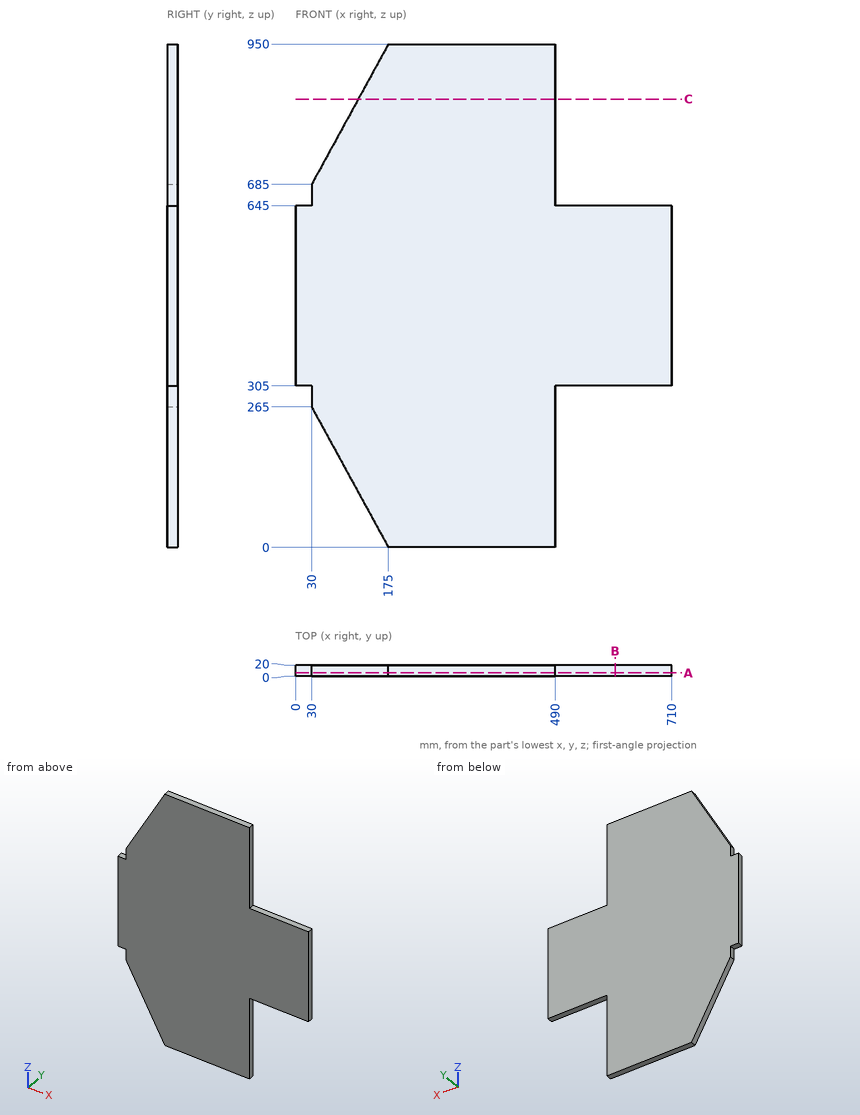
Geometry check sheet. Reference: drawing and pictorial views, mm from the part's lowest x, y, z. Give positions to 0.01 mm unless a question says otherwise; leave off trailing zeros. Write each loop counter-clockwise with the first axis right and the second up, starting at its lowest first coordinate (ties: lowest second). Pieces come first, ordered by that corner, then holes. Notation, with made-up numbers: (58, -35) - (89, -35) arc R16 cw to (89, -9) - close; hole circle Ø4 at (89, -12). An arc over 180 degrees is marked (long way). Use a Markdown table: item, result.
Q1. Section check A-A, the plane y = 6. Enter the section's corners in (x, z), then the cut area to 3 significant figures.
Computed:
| item | result |
|---|---|
| outline | (0, 305) - (30, 305) - (30, 265) - (175, 0) - (490, 0) - (490, 305) - (710, 305) - (710, 645) - (490, 645) - (490, 950) - (175, 950) - (30, 685) - (30, 645) - (0, 645) - close |
| area | 484,000 mm² |
Q2. Section check C-C, the plane z = 846. Enter the section's corners in (x, y), then the cut area to 3 significant figures.
Computed:
| item | result |
|---|---|
| outline | (118.09, 0) - (490, 0) - (490, 20) - (118.09, 20) - close |
| area | 7,440 mm² |
Q3. Thickness scan on L1, parallel to X at y = 5.75, z = 301; L2, parallel to Z at x = 652.5, y = 6.75; L3, parallel to X at y = 3.75, z = 236. Record the ranges inside material, lowest first. Write a range as [from, to].
Computed:
| item | result |
|---|---|
| L1 | x = [30, 490] |
| L2 | z = [305, 645] |
| L3 | x = [45.87, 490] |
Q4. Go/stop test with flat-tipped pins: P1, Ø12, axis at y = 15.5, z = 725.5, coming from the -X side; P2, Ø4, axis at y = 17, z = 223, coming from the +X side; P3, Ø1, axis at x = 378.5, z = 146.5, coming from the -Y side; P4, Ø10, axis at x = 597.5, y = 9, coming from the +Z side. Record where each tip stops, or that it passes through.
Computed:
| item | result |
|---|---|
| P1 | stops at x = 48.88 |
| P2 | stops at x = 490 |
| P3 | stops at y = 0 |
| P4 | stops at z = 645 |
Q5. Section check B-B, the plane x = 603. Enter the section's corners in (y, z).
Computed:
| item | result |
|---|---|
| outline | (0, 305) - (20, 305) - (20, 645) - (0, 645) - close |
